Could you check a few things on this model? Use its own coordinates, in mm. A direction names the side the tool comes from. Give positions to 0.01 mm unless a question says otherwise; leave off trailing zeros. Write each loop counter-clockwise with the first axis right and the second up, starting at its lowest first coordinate (ties: lowest second). Pieces come first, ordered by that corner, then holes. Notation, with made-up numbers: M -13,-7 L 7,-7 A29 cw 7,17 Z; hole C -4,-9.75 d6. An arc over 180 degrees is marked long. Write each question's results on one line, items separated by ' | '. Start each with the question number.
from build123d import *

# Parameters (mm, degrees)
SKETCH1_R           = 19.05
SKETCH1_R_2         = 9.525
BOSS_EXTRUDE1_DEPTH = 19.05
SKETCH1_3_R         = 19.05
SKETCH1_3_R_2       = 9.525
BOSS_EXTRUDE2_DEPTH = 25.4
SKETCH1_4_W         = 101.6
SKETCH1_4_H         = 12.7
BOSS_EXTRUDE3_DEPTH = 38.1
SKETCH2_W           = 82.55
SKETCH2_H           = 19.05
SKETCH3_W           = 50.8
SKETCH3_H           = 9.525


with BuildPart() as part:
    # Sketch1 → Boss-Extrude1 (new body)
    with BuildSketch(Plane.XY):
        with Locations((0, 63.5)):
            Circle(SKETCH1_R)
        with Locations(Location((0, 63.5, 0), (0, 0, 180))):
            Circle(SKETCH1_R_2, mode=Mode.SUBTRACT)
        with BuildLine():
            Line((-18.229762203, 69.029762203), (-23.759524406, 50.8))
            Line((-23.759524406, 50.8), (-28.575, 34.925))
            Line((-28.575, 34.925), (28.575, 34.925))
            Line((28.575, 34.925), (23.759524406, 50.8))
            Line((23.759524406, 50.8), (18.229762203, 69.029762203))
            ThreePointArc((18.229762203, 69.029762203), (18.84382485, 66.295132379), (19.05, 63.5))
            ThreePointArc((19.05, 63.5), (-2.795132379, 44.65617515), (-18.229762203, 69.029762203))
        make_face()
        with BuildLine():
            Line((-50.8, 41.275), (-50.8, 12.7))
            Line((-50.8, 12.7), (50.8, 12.7))
            Line((50.8, 12.7), (50.8, 41.275))
            ThreePointArc((50.8, 41.275), (48.010192091, 48.010192091), (41.275, 50.8))
            Line((41.275, 50.8), (23.759524406, 50.8))
            Line((23.759524406, 50.8), (28.575, 34.925))
            Line((28.575, 34.925), (-28.575, 34.925))
            Line((-28.575, 34.925), (-23.759524406, 50.8))
            Line((-23.759524406, 50.8), (-41.275, 50.8))
            ThreePointArc((-41.275, 50.8), (-48.010192091, 48.010192091), (-50.8, 41.275))
        make_face()
    extrude(amount=BOSS_EXTRUDE1_DEPTH)

    # Sketch1_3 → Boss-Extrude2 (add)
    with BuildSketch(Plane.XY):
        with BuildLine():
            Line((-18.229762203, 69.029762203), (-23.759524406, 50.8))
            Line((-23.759524406, 50.8), (-28.575, 34.925))
            Line((-28.575, 34.925), (28.575, 34.925))
            Line((28.575, 34.925), (23.759524406, 50.8))
            Line((23.759524406, 50.8), (18.229762203, 69.029762203))
            ThreePointArc((18.229762203, 69.029762203), (18.84382485, 66.295132379), (19.05, 63.5))
            ThreePointArc((19.05, 63.5), (-2.795132379, 44.65617515), (-18.229762203, 69.029762203))
        make_face()
        with Locations((0, 63.5)):
            Circle(SKETCH1_3_R)
        with Locations(Location((0, 63.5, 0), (0, 0, 180))):
            Circle(SKETCH1_3_R_2, mode=Mode.SUBTRACT)
    extrude(amount=BOSS_EXTRUDE2_DEPTH)

    # Sketch1_4 → Boss-Extrude3 (add)
    with BuildSketch(Plane.XY):
        with Locations((0, 6.35)):
            Rectangle(SKETCH1_4_W, SKETCH1_4_H)
    extrude(amount=BOSS_EXTRUDE3_DEPTH)

    # Sketch2 → Loft1 section 0
    with BuildSketch(Plane.XY.offset(19.05)):
        with Locations((0, 34.925)):
            Rectangle(SKETCH2_W, SKETCH2_H)
    # Sketch3 → Loft1 section 1
    with BuildSketch(Plane.XY.offset(44.45)):
        with Locations((0, 30.1625)):
            Rectangle(SKETCH3_W, SKETCH3_H)
    loft()


solid = part.part
Q1. If we section it at A-A (z = 3): Please give me the cut outline in (x, y) (3 decimals), plus the area to 3 significant figures.
Q2. If we mould it in two halves opening along Y, with no side actions, what happens to faces 4 (the face through (48.08, 47.94, 9.39)), 5 (the face through (-1, 12.7, 28)), 6 (the face through (-1, 0, 19))? For each: pulls with the +Y half, pulls with the -Y half, needs draft (parallel to the pull), parting line crosses it, or undercut.
Q3. If we section it at C-C (z = 24): Count the separate pieces of the cut face and the enclosed holes in it, plus the area to 3 significant figures.
Q4. Please list where these lines run through material, in increasing order: line 1 (Y direction, x = 0, z = 18) (3 decimals); line 2 (Z direction, x = -11, y = 15.5); line 3 (Y direction, x = 35, z = 12). Write a range as [from, to].
Q5. For faces 1 (the face through (-1, 6, 38.1)), 2 (the face through (-32, 50.8, 9)), 3 (the face through (-0.4, 53.6, 25.4)), which set-ups out of +Z, -Z, +X, -X, +Y, -Y let a thin tool reach every point of the face, with its end or its side?
Q6. If we section it at B-B (y = 63.5): Please give me the cut outline in (x, z) (3 decimals).
Q7. I'm going to push flat-ended pins straight in: P1, Ø4, axis at x = -11.5, y = 6.5, coming from the +Z side; P2, Ø2, axis at x = -38, y = 18.5, coming from the +Z side; P3, Ø14, axis at x = -32, z = 8.5, coming from the +Y side; P4, Ø15, axis at x = 0, y = 63.5, coming from the +Z side. Where does each tip first touch, or does it pass through?
Determined:
1) outline: M -50.8,0 L 50.8,0 L 50.8,41.275 A9.525 ccw 41.275,50.8 L 23.76,50.8 L 18.23,69.03 A19.05 ccw -18.23,69.03 L -23.76,50.8 L -41.275,50.8 A9.525 ccw -50.8,41.275 Z; hole C 0,63.5 d19.05 | area: 5,970 mm²
2) face 4: pulls with the +Y half | face 5: undercut | face 6: pulls with the -Y half
3) separate pieces: 2 | enclosed holes: 1 | area: 3,860 mm²
4) line 1: y = [0, 53.975], [73.025, 82.55] | line 2: z = [0, 19.05] | line 3: y = [0, 50.8]
5) face 1: +Z, +X, -X, -Y | face 2: +Z, -Z, -X, +Y | face 3: +Z, +X, -X, +Y
6) outline: M -19.907,0 L -9.525,0 L -9.525,25.4 L -19.907,25.4 Z; M 9.525,0 L 19.907,0 L 19.907,25.4 L 9.525,25.4 Z
7) P1: stops at z = 38.1 | P2: stops at z = 19.05 | P3: stops at y = 50.8 | P4: passes through
